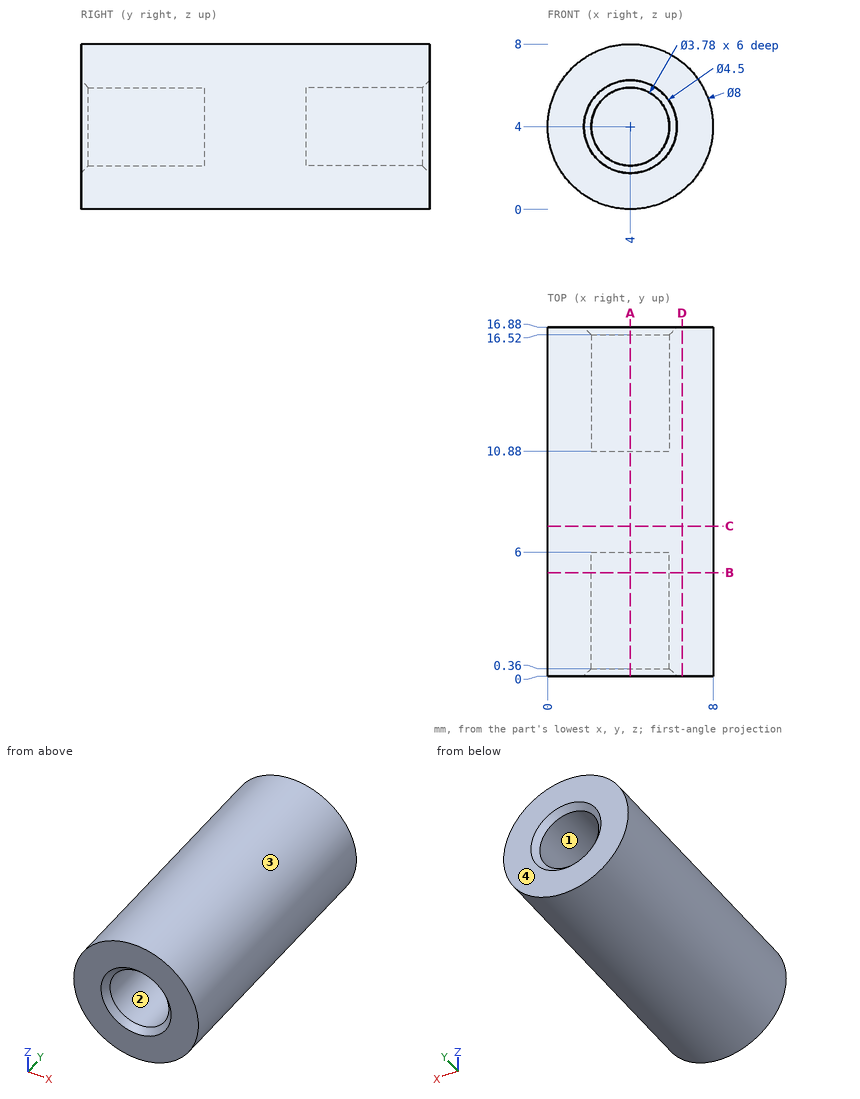
Answer from the drawing. Dimensions are ordinates in mm from the lowest x, y and z of the part. Give positions to 0.01 mm unless a question says otherwise; leave off trailing zeros. Order: outer loops, then holes, each group sorted by start corner. A loop starts at its lowest first (then second) coordinate and runs counter-clockwise, first axis right, second up. Notation, with made-up numbers: (62.5, 32.5) -> (105.5, 32.5) arc R18 ccw to (105.5, 55.5) -> close; hole circle Ø9 at (66, -15). An arc over 180 degrees is marked (long way). One line per item, written item: value. Start each with the question number.
(1) The part is cut by section C-C (y = 7.25). Determine the outline of the cut face in (x, z).
(2) The part is cut by section B-B (y = 5). Determine the outline of the cut face in (x, z).
(3) For a pull along Z with two mould halves and no side action, classify the marked faces 1, 2, 3 and 4 as released by +Z, released by -Z, zero draft, split by the parting line, or undercut.
(4) Straight lines are drawn through the part: L1, parallel to Z at x = 4, y = 12; L2, parallel to Z at x = 5.25, y = 1. For each, find the intervals that lie inside material, in ascending order.
(5) The part is cut by section D-D (x = 6.5). Determine the outline of the cut face in (y, z), and give its area (3 significant figures).
(6) The part is cut by section A-A (x = 4). Determine the outline of the cut face in (y, z), and give its area (3 significant figures).
(7) Flat-ended cylindrical pins translate along their axes: P1, Ø2, axis at y = 7.5, z = 2.5, coming from the -X side; P2, Ø1, axis at y = 11, z = 2.5, coming from the -X side; P3, Ø3.5, axis at x = 4, z = 4, coming from the -Y side. Find the tip coordinate at first contact, or state that the pin passes through.
Taken from the geometry:
1. outline: circle Ø8 at (4, 4)
2. outline: circle Ø8 at (4, 4); hole circle Ø3.78 at (4, 4)
3. face 1: undercut
3. face 2: undercut
3. face 3: split by the parting line
3. face 4: zero draft
4. L1: 0 to 2.11, 5.89 to 8
4. L2: 0.2 to 2.58, 5.42 to 7.8
5. outline: (0, 0.88) -> (16.88, 0.88) -> (16.88, 7.12) -> (0, 7.12) -> close
5. area: 105 mm^2
6. outline: (0, 0) -> (16.88, 0) -> (16.88, 1.75) -> (16.52, 2.11) -> (10.88, 2.11) -> (10.88, 5.89) -> (16.52, 5.89) -> (16.88, 6.25) -> (16.88, 8) -> (0, 8) -> (0, 6.25) -> (0.36, 5.89) -> (6, 5.89) -> (6, 2.11) -> (0.36, 2.11) -> (0, 1.75) -> close
6. area: 89.4 mm^2
7. P1: x = 0.03
7. P2: x = 0.13
7. P3: y = 6
